For this review, take the finished solid that the model builds, in its own axes (mm). Give positions to 0.01 mm unless a question says otherwise; leave off trailing zeros. Use CSV: the item, a comma, the result in double quotes. Start each with the question number.
1. Wall thickness on line 1 (Z direction, x = -0.5, y = 2.25); line 2 (X direction, y = -2.75, z = 119); line 3 (Z direction, x = 24, y = -7.75): over which ranges is each line inside the solid? List them lowest first.
2. Mouldability with a two-part tool opening along Y and no side actions: class faces 1 (the flat face through (17, 12.7, 105)), 2 (the flat face through (17, -12.7, 105)) as pulls with the +Y half, pulls with the -Y half, needs draft (parallel to the pull), parting line crosses it, or undercut.
3. For pin 1 (10 mm diameter, centred on x = 40, y = -2, fed in from +Z); pin 2 (8 mm diameter, centred on x = 70.5, y = -5.5, fed in from +Z); pin 3 (5 mm diameter, centred on x = 57.5, y = 4.5, fed in from -Z), all flat-tipped, find the tip position at first contact; note any pin that passes through.
```python
from build123d import *

# Parameters (mm, degrees)
F1_DEPTH = 12.7
F1_TAPER = -3


with BuildPart() as f1:
    # F0 (on Front) → F1 (new body, symmetric)
    with BuildSketch(Plane.XZ):
        Polygon((147.9144990444, 156.5441638231), (-119.0584152937, 156.5441638231), (-116.1468625069, 49.0151830018), (147.9144990444, 49.0151830018), align=None)
    extrude(amount=F1_DEPTH, both=True, taper=F1_TAPER)


solid = f1.part
```
Check result:
1,line 1,"z = 48.9 to 156.66"
1,line 2,"x = -118.19 to 148.06"
1,line 3,"z = 48.61 to 156.95"
2,face 1,"pulls with the +Y half"
2,face 2,"pulls with the -Y half"
3,pin 1,"stops at z = 156.91"
3,pin 2,"stops at z = 157.04"
3,pin 3,"stops at z = 48.65"
